Part print with two shaded views. Sizes in mm from the minimum x, y, z corner. Coordinates: 2 decimals unless noted, no trailing zeros. Loops run counter-clockwise (first coordinate to the right, second up) from the corner with the lowest first, then second, coordinate; pieces in that order, holes last. Notation, with made-up numbers: (41, 14) -> (68, 14) arc R6 cw to (68, 19) -> close; hole circle Ø3 at (-2, 72.5). An arc over 180 degrees is marked (long way). Answer as a JSON object with one key per item and string values. Group by question number.
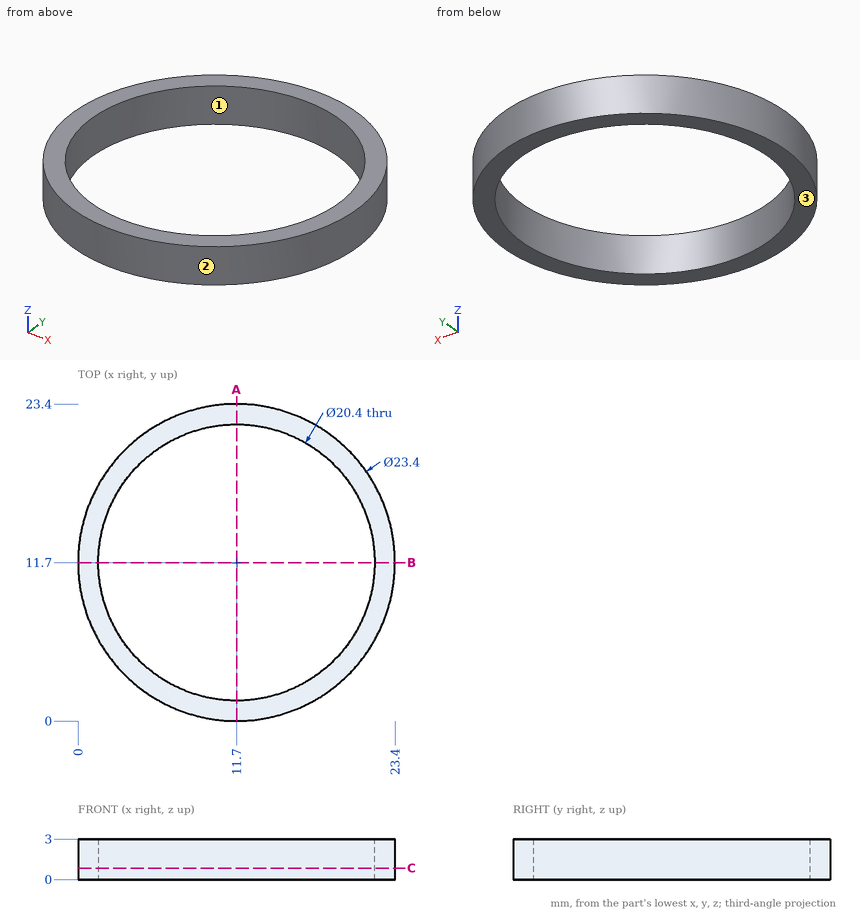
Item 1: Band-saw the part on A-A, the plane x = 11.7. List the corners of the cut face in (y, z), and give its area (3 significant figures).
Item 2: Pull direction X, two halves, no side cores. Call the marked faces 1, 2 and 3: +X half, -X half, draft (parallel to the pull), parting line (faces both ways), or undercut.
Item 3: Band-saw the part on C-C, the plane z = 0.85. List the corners of the cut face in (x, y), and give its area (3 significant figures).
Item 4: Drill centre lines: L1, parallel to X at y = 11.5, z = 0.5; L2, parallel to X at y = 13, z = 0.25. Where is each one in solid material? Low to high.
Item 5: Flat gauge pins, fed straight in: P1, Ø1, axis at x = 19, y = 5.5, coming from the -Z side; P2, Ø1.5, axis at y = 16.5, z = 1.5, coming from the -X side; P3, Ø1.5, axis at x = 19, z = 0.5, coming from the +Y side; P4, Ø6, axis at x = 18, y = 6, coming from the +Z side. Where does each tip first touch, or does it go through?
Reply:
{
 "1": {"outline": "(0, 0) -> (1.5, 0) -> (1.5, 3) -> (0, 3) -> close; (21.9, 0) -> (23.4, 0) -> (23.4, 3) -> (21.9, 3) -> close", "area": "9.00 mm²"},
 "2": {"face 1": "undercut", "face 2": "parting line", "face 3": "draft"},
 "3": {"outline": "circle Ø23.4 at (11.7, 11.7); hole circle Ø20.4 at (11.7, 11.7)", "area": "103 mm²"},
 "4": {"L1": "0 to 1.5, 21.9 to 23.4", "L2": "0.07 to 1.58, 21.82 to 23.33"},
 "5": {"P1": "through", "P2": "x = 0.72", "P3": "y = 21.39", "P4": "z = 3"}
}
